CAD build for the part. Positions are in the model's coordinates, mm. A direction names the side the tool comes from. Round coordinates to 2 decimals unless told otherwise and drop trailing zeros. Loops run counter-clockwise (first coordinate to the right, second up) from the corner with the lowest first, then second, coordinate; pieces in that order, holes last.
from build123d import *

# Parameters (mm, degrees)
SKETCH1_R            = 127
BOSS_EXTRUDE1_DEPTH  = 3.175
M5_CLEARANCE_HOLE1_D = 5.5
CIRPATTERN1_COUNT    = 6
BOSS_EXTRUDE2_DEPTH  = 3.175
CIRPATTERN2_COUNT    = 6
CUT_EXTRUDE1_DEPTH   = 286.374530912


with BuildPart() as part:
    # Sketch1 → Boss-Extrude1 (new body)
    with BuildSketch(Plane.XY):
        Circle(SKETCH1_R)
    extrude(amount=BOSS_EXTRUDE1_DEPTH)

    # M5 Clearance Hole1 (through all)
    with Locations(Plane(origin=(0, 0, 0), x_dir=(-1, 0, 0), z_dir=(0, 0, -1))):
        with Locations((-58.2494214, 58.493652703), (-82.549819355, -0.172697611), (-93.238867767, 66.113565457), (-112.679186132, 19.180485205), (-11.733270063, 4.860079591), (-68.767621753, 45.667457762), (-80.917820731, 16.334282605), (-35.199810189, 14.580238773)):
            m5_clearance_hole1 = Hole(M5_CLEARANCE_HOLE1_D / 2)

    # CirPattern1: M5 Clearance Hole1 ×6 about axis
    cirpattern1_axis = Axis((-0.255716285, -0.105921153, 0), (0, 0, 1))
    for i in range(1, CIRPATTERN1_COUNT):
        add(m5_clearance_hole1.rotate(cirpattern1_axis, i * 360 / CIRPATTERN1_COUNT), mode=Mode.SUBTRACT)

    # Sketch6 → Boss-Extrude2 (add)
    with BuildSketch(Plane(origin=(0, 0, 0), x_dir=(-1, 0, 0), z_dir=(0, 0, -1))):
        with BuildLine():
            Line((-97.979344732, 78.730580539), (-147.8457425, 99.385918801))
            ThreePointArc((-147.8457425, 99.385918801), (-169.716100659, 99.385918801), (-185.180779221, 83.92124024))
            Line((-185.180779221, 83.92124024), (-200.976037892, 45.788112535))
            Line((-200.976037892, 45.788112535), (-124.709782483, 14.197595193))
            Line((-124.709782483, 14.197595193), (-97.979344732, 78.730580539))
        make_face()
    boss_extrude2 = extrude(amount=-BOSS_EXTRUDE2_DEPTH)

    # CirPattern2: Boss-Extrude2 ×6 about axis
    cirpattern2_axis = Axis((0, 0, 0), (0, 0, 1))
    for i in range(1, CIRPATTERN2_COUNT):
        add(boss_extrude2.rotate(cirpattern2_axis, i * 360 / CIRPATTERN2_COUNT))

    # Sketch7 → Cut-Extrude1 (cut, through all)
    with BuildSketch(Plane.XY.offset(3.175)):
        Polygon((7.292181047, -0.766439112), (4.309846265, 5.931994479), (-2.982334782, 6.698433592), (-7.292181047, 0.766439112), (-4.309846265, -5.931994479), (2.982334782, -6.698433592), align=None)
    extrude(amount=-CUT_EXTRUDE1_DEPTH, mode=Mode.SUBTRACT)


solid = part.part
Item 1: Mould opens along Y. For faces 1 (the cylindrical face through (48.503, -117.373, 1.565)), 2 (the cylindrical face through (-170.886, 96.974, 1.565)), 3 (the cylindrical face through (-48.503, 117.373, 1.565)), 4 (the flat face through (-55.62, -157.35, 1.57)) say: released by +Y, released by -Y, zero draft, split by the parting line, or undercut.
Verdict:
face 1: released by -Y
face 2: undercut
face 3: released by +Y
face 4: undercut
Item 2: Cut at A-A (z = 1.35). State how many separate pieces and enclosed holes the cut face has, plus the area to 3 significant figures.
Verdict:
separate pieces: 1
enclosed holes: 49
area: 81,000 mm2
Item 3: Wall check: L1, parallel to X at y = -5, z = 1.45; L2, parallel to X at y = -39.5, z = 0.35; L3, parallel to Y at x = -7, z = 0.5. Give the ranges that are in metal, low to high.
Verdict:
L1: x = -126.9 to -14.99, -9.5 to -4.72, 4.22 to 126.9
L2: x = -185.8 to -7.66, -2.87 to 72.76, 75.03 to 120.7
L3: y = -201.06 to -40.29, -36.02 to 0.11, 1.17 to 80.33, 84.78 to 190.71
Item 4: 3-axis set-ups, long thin cutter, end or side, ignore diameter. For faces 5 (the flat face through (108.458, -126.845, 1.565)), 6 (the flat face through (55.62, 157.35, 1.57)), 7 (the cylindrical face through (-77.4, -100.69, 1.57)), 8 (the flat face through (-108.458, 126.845, 1.565)): which of +Z, -Z, +X, -X, +Y, -Y reach the whole face in a straight line?
Verdict:
face 5: +Z, -Z, -Y
face 6: +Z, -Z, +X
face 7: +Z, -Z
face 8: +Z, -Z, +Y
Item 5: Cut at B-B (y = -158). List the corners of the cut face in (x, z) (3 decimals), plus the area to 3 significant figures.
Verdict:
outline: (-55.707, 0) - (14.746, 0) - (14.746, 3.175) - (-55.707, 3.175) - close
area: 224 mm2
Item 6: Flat gauge pin, fed straight in: P1, Ø9, axis at x = 1.44, y = 12.76, coming from the -Z side. Where does the tip first touch, or does it go through?
Verdict:
P1: stops at z = 0
